Source: three-view drawing plus pictorial views. Frame: mm from the lowest corner of the part. Give positions to 0.01 mm unless a question says otherwise; leave off trailing zeros. Order: outer loops, then holes, each group sorted by start corner. A loop starts at its lowest first (then second) coordinate and runs counter-clockwise, first axis right, second up. Notation, with made-up numbers: M 4,70.25 L 54,70.25 A35 ccw 54,109.25 Z; hole C 2,47.5 d4. An arc over 180 degrees is marked long. Use CSV: the item, a comma, the result in double quotes.
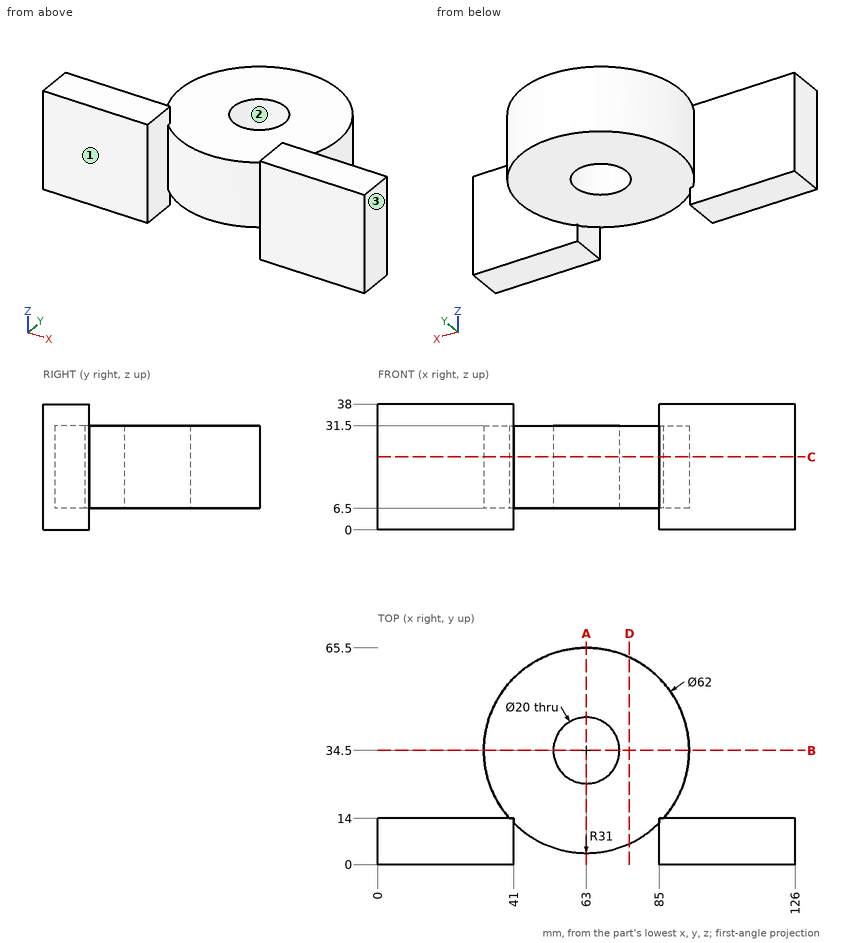
1. Line query: line 1 (Y direction, x = 63, z = 20.5); line 2 (X direction, y = 34, z = 23); line 3 (Y direction, x = 109, z = 28). Output: solid intervals per line, ascending.
Answer:
line 1,"3.5 to 24.5, 44.5 to 65.5"
line 2,"32 to 53.01, 72.99 to 94"
line 3,"0 to 14"
2. Pull-direction query (X, two-part tool) for the marked faces 1, 2 and 3; classes: +X half, -X half, draft (parallel to the pull), parting line (faces both ways), or undercut.
Answer:
face 1,"draft"
face 2,"undercut"
face 3,"+X half"
3. Pin query (flat end, axial travel): pin 1 Ø19 at (x, z) = (30.5, 18.5) entering from +Y; pin 2 Ø19 at (x, z) = (98.5, 14) entering from +Y; pin 3 Ø8 at (x, y) = (60, 32.5) entering from -Z; pin 4 Ø4 at (y, z) = (32.5, 16.5) entering from +X. Return the tip coordinate at first contact, or that it passes through.
Answer:
pin 1,"y = 55.28"
pin 2,"y = 51.38"
pin 3,"through"
pin 4,"x = 94"
4. Section C-C, the plane z = 22. Return the cut outline in (x, y).
Answer:
outline,"M 0,0 L 41,0 L 41,12.66 A31 ccw 85,12.66 L 85,0 L 126,0 L 126,14 L 86.25,14 A31 ccw long 39.75,14 L 0,14 Z; hole C 63,34.5 d20"
5. Section B-B, the plane y = 34.5. Return the cut outline in (x, z), plus the area to 3 significant figures.
Answer:
outline,"M 32,6.5 L 53,6.5 L 53,31.5 L 32,31.5 Z; M 73,6.5 L 94,6.5 L 94,31.5 L 73,31.5 Z"
area,"1,050 mm2"
6. Section D-D, the plane x = 76. Return the cut outline in (y, z).
Answer:
outline,"M 6.36,6.5 L 62.64,6.5 L 62.64,31.5 L 6.36,31.5 Z"
7. Section A-A, the plane x = 63. Return the cut outline in (y, z), plus the area to 3 significant figures.
Answer:
outline,"M 3.5,6.5 L 24.5,6.5 L 24.5,31.5 L 3.5,31.5 Z; M 44.5,6.5 L 65.5,6.5 L 65.5,31.5 L 44.5,31.5 Z"
area,"1,050 mm2"
